from build123d import *

# Parameters (mm, degrees)
F4_W      = 2
F4_H      = 4
F6_R      = 1.5
F7_DEPTH  = 12.5
F8_R      = 1.5
F9_DEPTH  = 12.5
F10_R     = 1.5
F11_DEPTH = 12.5


with BuildPart() as f2:
    # F0 (on Front) → F2 (revolve)
    with BuildSketch(Plane.XZ):
        with BuildLine():
            Line((-107.5, 0), (0, 0))
            Line((0, 0), (0, 67))
            ThreePointArc((0, 67), (-63.47382, 49.101651), (-107.5, 0))
        make_face()
    revolve(axis=Axis((0, 0, 33.5), (0, 0, 1)))

    # F1 (on Front) → F3 (revolve, cut)
    with BuildSketch(Plane.XZ):
        with BuildLine():
            Line((-105.5, 0), (0, 0))
            Line((0, 0), (0, 65))
            ThreePointArc((0, 65), (-61.789194, 47.171307), (-105.5, 0))
        make_face()
    revolve(axis=Axis((0, 0, 32.5), (0, 0, 1)), mode=Mode.SUBTRACT)

    # F4 (on Front) → F5 (revolve)
    with BuildSketch(Plane.XZ):
        with Locations((-106.5, -2)):
            Rectangle(F4_W, F4_H)
    revolve(axis=Axis((0, 0, -3.064933), (0, 0, -1)))

    # F6 (on Front) → F7 (join, symmetric)
    with BuildSketch(Plane.XZ):
        Polygon((-106.584328, 26.365628), (-93.438419, 19.129254), (-84.525248, 31.514426), align=None)
        with Locations((-95.591055, 24.988731)):
            Circle(F6_R, mode=Mode.SUBTRACT)
    extrude(amount=F7_DEPTH, both=True)

    # F8 (on Front) → F9 (join, symmetric)
    with BuildSketch(Plane.XZ):
        Polygon((84.52525, 31.514422), (93.43842, 19.12925), (106.584329, 26.365624), align=None)
        with Locations((95.591056, 24.988727)):
            Circle(F8_R, mode=Mode.SUBTRACT)
    extrude(amount=F9_DEPTH, both=True)

    # F10 (on Front) → F11 (join, symmetric)
    with BuildSketch(Plane.XZ):
        with BuildLine():
            ThreePointArc((8, 65.735355), (0, 72.135355), (-8, 65.735355))
            Line((-8, 65.735355), (8, 65.735355))
        make_face()
        with Locations((0, 69.362663)):
            Circle(F10_R, mode=Mode.SUBTRACT)
    extrude(amount=F11_DEPTH, both=True)


solid = f2.part
Can you work these out from the model? Positions are in its coordinate system, mm. A direction names the side the tool comes from. Round coordinates to 2 decimals unless told otherwise and drop trailing zeros. Use CSV: the item, a comma, the result in double quotes.
(1) I need wall thicknesses on line 1 along Y through (x, z) = (0, -2.95); line 2 along X through (y, z) = (12.5, 15.5). Which ranges of each line are inside material? Lowest first, please.
Check values:
line 1,"-107.5 to -105.5, 105.5 to 107.5"
line 2,"-97.74 to -95.14, 95.14 to 97.74"
(2) We'd pull the mould along Z, two halves only. Please class faces 1 (the flat face through (-96, 12.5, 27)), 2 (the cylindrical face through (0.148, -0.175, 72.134)), 3 (the flat face through (100.528, -0.175, 23.032)): +Z half, -Z half, draft (parallel to the pull), parting line (faces both ways), or undercut.
Check values:
face 1,"draft"
face 2,"+Z half"
face 3,"undercut"
(3) On a 3-axis mill with a long thin cutter (end or side, diameter ignored), from which of +Z, -Z, +X, -X, +Y, -Y can I reach the whole of each face in a straight line? I mean faces 4 (the flat face through (95, -12.5, 27)), 5 (the flat face through (95, 12.5, 27)), 6 (the flat face through (-96, -12.5, 27)). Say none if no direction works.
Check values:
face 4,"+Z, +X, -Y"
face 5,"+Z, +X, +Y"
face 6,"+Z, -X, -Y"
(4) I'm going to push flat-ended pins straight in: pin 1 (12 mm diameter, centred on y = -67.5, z = 4.5, fed in from -X); pin 2 (2.5 mm diameter, centred on x = 0, z = 69.36, fed in from -Y); pin 3 (1 mm diameter, centred on y = 7.5, z = 24.5, fed in from -X); pin 4 (10 mm diameter, centred on x = -17.5, y = 68, fed in from +Z). Where does each tip first touch, or does it pass through?
Check values:
pin 1,"x = -86.79"
pin 2,"through"
pin 3,"x = -104.1"
pin 4,"z = 47.99"
